Part model, mm, in its own coordinate system. A direction names the side the tool comes from. Give positions to 0.01 mm unless a question says otherwise; leave off trailing zeros. Order: outer loops, then holes, each group sorted by start corner. A loop starts at its lowest first (then second) coordinate and runs counter-clockwise, first axis right, second up. Notation, with made-up numbers: (85, 31.5) - (114, 31.5) arc R16 ccw to (114, 44.5) - close; hole circle Ø2 at (89.5, 0.5). An arc over 180 degrees is marked (long way). One line per item, written item: value.
```python
from build123d import *

# Parameters (mm, degrees)
SALIENTE_EXTRUIR1_DEPTH = 5
CROQUIS2_W              = 13
CROQUIS2_H              = 3
SALIENTE_EXTRUIR2_DEPTH = 16
CROQUIS3_R              = 2
CORTAR_EXTRUIR1_DEPTH   = 16
CROQUIS7_R              = 2
CORTAR_EXTRUIR2_DEPTH   = 16


with BuildPart() as part:
    # Croquis1 → Saliente-Extruir1 (new body)
    with BuildSketch(Plane(origin=(0, 0, 0), x_dir=(1, 0, 0), z_dir=(0, 1, 0))):
        Polygon((27.5, -11.160546845), (-12.5, -11.160546845), (-12.5, -16.760546845), (-25.5, -16.760546845), (-25.5, -1.160546845), (9.5, -1.160546845), (9.5, 35.839453155), (27.5, 35.839453155), align=None)
    extrude(amount=SALIENTE_EXTRUIR1_DEPTH)

    # Croquis2 → Saliente-Extruir2 (add)
    with BuildSketch(Plane(origin=(0, 0, 0), x_dir=(-1, 0, 0), z_dir=(0, -1, 0))):
        with Locations((19, -15.260546845)):
            Rectangle(CROQUIS2_W, CROQUIS2_H)
    extrude(amount=SALIENTE_EXTRUIR2_DEPTH)

    # Croquis3 → Cortar-Extruir1 (cut)
    with BuildSketch(Plane(origin=(0, 5, 0), x_dir=(1, 0, 0), z_dir=(0, 1, 0))):
        with Locations(Location((16.5, 31.339453155, 0), (0, 0, 270))):
            Circle(CROQUIS3_R)
        with Locations(Location((16.5, 21.339453155, 0), (0, 0, 270))):
            Circle(CROQUIS3_R)
        with Locations(Location((16.5, 11.339453155, 0), (0, 0, 270))):
            Circle(CROQUIS3_R)
    extrude(amount=-CORTAR_EXTRUIR1_DEPTH, mode=Mode.SUBTRACT)

    # Croquis7 → Cortar-Extruir2 (cut)
    with BuildSketch(Plane(origin=(0, 0, 13.760546845), x_dir=(-1, 0, 0), z_dir=(0, 0, -1))):
        with Locations((20.5, -11)):
            Circle(CROQUIS7_R)
    extrude(amount=-CORTAR_EXTRUIR2_DEPTH, mode=Mode.SUBTRACT)


solid = part.part
```
1) Drop flat-ended pins along their axis: P1, Ø3, axis at y = -6.5, z = 14, coming from the +X side; P2, Ø4, axis at x = -5, y = 1.5, coming from the -Z side; P3, Ø3, axis at x = 16.5, z = -31.34, coming from the +Y side; P4, Ø4, axis at x = 15.5, y = 2.5, coming from the +Z side. Give the stop position or say it passes through.
Answer:
P1: stops at x = -12.5
P2: stops at z = 1.16
P3: passes through
P4: stops at z = 11.16
2) Slice it at A-A on y = -11. Write the cut outline in (x, z), then the cut area to 3 significant figures.
Answer:
outline: (-25.5, 13.76) - (-22.5, 13.76) - (-22.5, 16.76) - (-25.5, 16.76) - close; (-18.5, 13.76) - (-12.5, 13.76) - (-12.5, 16.76) - (-18.5, 16.76) - close
area: 27.0 mm2
3) Two-plate mould, pull along Z, no slides. Class faces 1 (the face through (-19, -8, 13.761)), 2 (the face through (18.186, 2.535, -30.264)), 3 (the face through (-19.026, -9.648, 15.24)): pulls with the +Z half, pulls with the -Z half, needs draft (parallel to the pull), parting line crosses it, or undercut.
Answer:
face 1: pulls with the -Z half
face 2: undercut
face 3: needs draft
4) Slice it at C-C on z = -21. Write the cut outline in (x, y).
Answer:
outline: (9.5, 0) - (14.53, 0) - (14.53, 5) - (9.5, 5) - close; (18.47, 0) - (27.5, 0) - (27.5, 5) - (18.47, 5) - close
5) Wall check: line 1 along Y through (x, z) = (-20.5, 15.85); line 2 along Y through (x, z) = (-17.5, 5); line 3 along Z through (x, y) = (-14.5, -12). Give the ranges that are in metal, low to high. Write a range as [from, to].
Answer:
line 1: y = [-16, -13], [-9, 5]
line 2: y = [0, 5]
line 3: z = [13.76, 16.76]
6) Which spindle directions (+Z, -Z, +X, -X, +Y, -Y) get a long thin tool onto all of the face, cutting with end or side? Do faces 4 (the face through (9.5, 2, -17)), 5 (the face through (18, 2, -35.839)), 6 (the face through (-12.5, -3, 15)). Say none if no direction does.
Answer:
face 4: -Z, -X, +Y, -Y
face 5: -Z, +X, -X, +Y, -Y
face 6: +Z, +X, +Y, -Y
7) Slice it at B-B on x = -20.5. Write the cut outline in (y, z).
Answer:
outline: (-16, 13.76) - (-13, 13.76) - (-13, 16.76) - (-16, 16.76) - close; (-9, 13.76) - (0, 13.76) - (0, 1.16) - (5, 1.16) - (5, 16.76) - (-9, 16.76) - close
8) Slice it at D-D on x = 16.5. Write the cut outline in (y, z), then the cut area to 3 significant figures.
Answer:
outline: (0, -35.84) - (5, -35.84) - (5, -33.34) - (0, -33.34) - close; (0, -29.34) - (5, -29.34) - (5, -23.34) - (0, -23.34) - close; (0, -19.34) - (5, -19.34) - (5, -13.34) - (0, -13.34) - close; (0, -9.34) - (5, -9.34) - (5, 11.16) - (0, 11.16) - close
area: 175 mm2
